Design review of the part shown in the three views and the two pictorial views. Dimensions are in mm from the part's minimum x, y and z. A direction names the side the tool comes from. Give positions to 0.01 mm unless a question says otherwise; leave off trailing zeros. Loops run counter-clockwise (first coordinate to the right, second up) from the corner with the lowest first, then second, coordinate; pieces in that order, holes last.
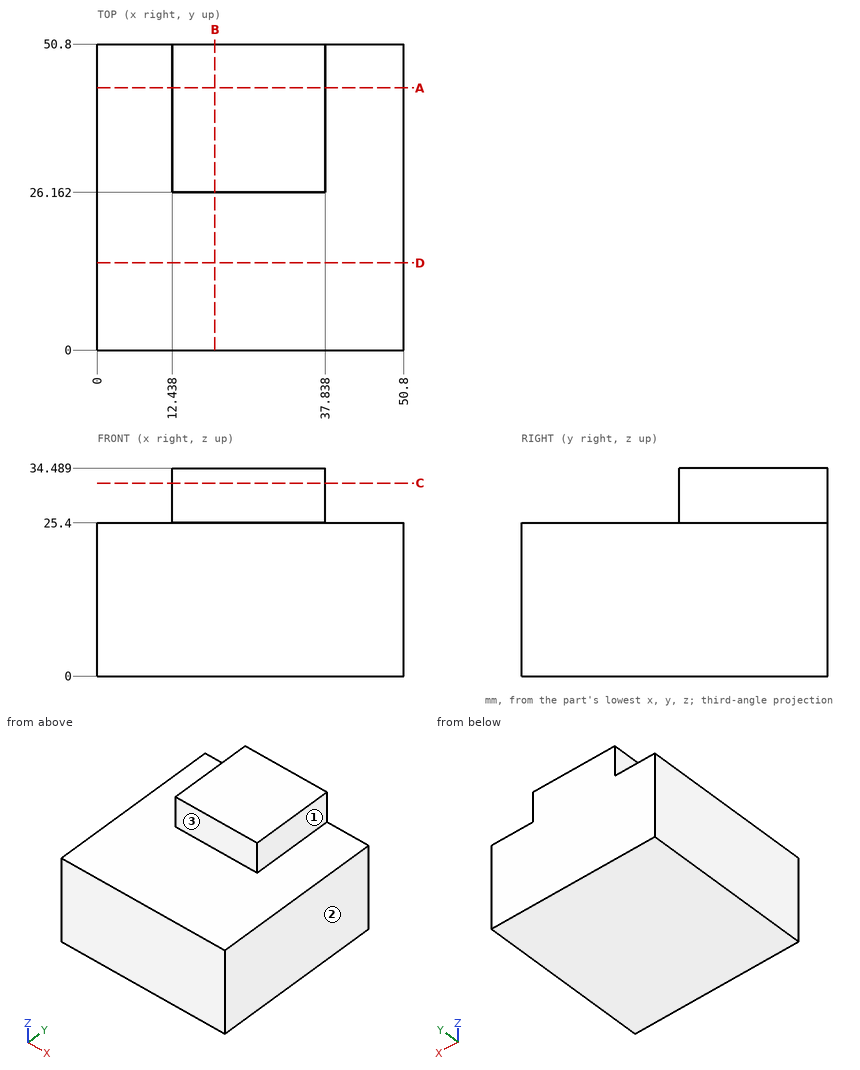
Q1. Machinability: for the marked faces 1, 2 and 3, which of the approach directions +Z, -Z, +X, -X, +Y, -Y give a long, thin tool a straight path to every point of the face, cutting with its end or side? Answer none if there is none.
Answers:
face 1: +Z, +X, +Y, -Y
face 2: +Z, -Z, +X, +Y, -Y
face 3: +Z, +X, -X, -Y
Q2. Consider section A-A on y = 43.5. Give the boundary of the cut face in (x, z), plus the area to 3 significant figures.
Answers:
outline: (0, 0) - (50.8, 0) - (50.8, 25.4) - (37.84, 25.4) - (37.84, 34.49) - (12.44, 34.49) - (12.44, 25.4) - (0, 25.4) - close
area: 1,520 mm2
Q3. For pin 1 Ø7.5 at (x, z) = (23.5, 28) entering from -Y; pin 2 Ø7.5 at (y, z) = (41.5, 31) entering from -X; pin 3 Ø10 at (x, y) = (35.5, 17.5) entering from +Z, all flat-tipped, find the tip position at first contact; note any pin that passes through.
Answers:
pin 1: stops at y = 0
pin 2: stops at x = 12.44
pin 3: stops at z = 25.4
Q4. Consider section D-D on y = 14.5. Give the boundary of the cut face in (x, z).
Answers:
outline: (0, 0) - (50.8, 0) - (50.8, 25.4) - (0, 25.4) - close
Q5. Consider section B-B on x = 19.5. Give the boundary of the cut face in (y, z), plus the area to 3 significant figures.
Answers:
outline: (0, 0) - (50.8, 0) - (50.8, 34.49) - (26.16, 34.49) - (26.16, 25.4) - (0, 25.4) - close
area: 1,510 mm2
Q6. For probe 1 along Z at (x, y) = (45, 19); probe 2 along Y at (x, z) = (35.5, 28.5); probe 3 along X at (y, z) = (41, 27.5), list the stretches that pass through material, from the lowest coordinate up.
Answers:
probe 1: z = 0 to 25.4
probe 2: y = 26.16 to 50.8
probe 3: x = 12.44 to 37.84
Q7. Consider section C-C on z = 32. Give the boundary of the cut face in (x, y).
Answers:
outline: (12.44, 26.16) - (37.84, 26.16) - (37.84, 50.8) - (12.44, 50.8) - close
